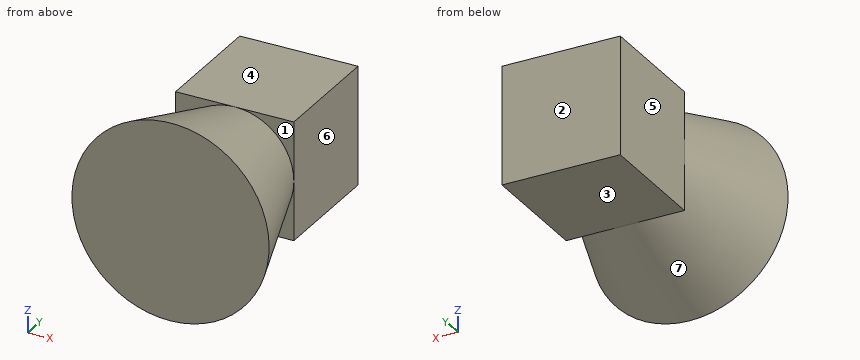
```python
from build123d import *

# Parameters (mm, degrees)
SKETCH_2_W      = 30
SKETCH_2_H      = 30
EXTRUDE_1_DEPTH = 30


with BuildPart() as part:
    # 草图2 → 凸台-拉伸1 (new body)
    with BuildSketch(Plane(origin=(0, 0, 0), x_dir=(1, 0, 0), z_dir=(0, 1, 0))):
        Rectangle(SKETCH_2_W, SKETCH_2_H)
    extrude(amount=EXTRUDE_1_DEPTH)

    # 草图3 → 旋转1 (revolve)
    with BuildSketch(Plane.XY, mode=Mode.PRIVATE) as revolve_1_sk:
        Polygon((0, 0), (15, 0), (25, -30), (0, -30), align=None)
    revolve(revolve_1_sk.sketch.rotate(Axis((0, -30, 0), (0, 1, 0)), 90), axis=Axis((0, -30, 0), (0, 1, 0)))


solid = part.part
```
Geometry check sheet. Reference: the model listing, model coordinates, mm. Face numbers are marked on the shaded views. A direction names the side the tool comes from. Round coordinates to 2 decimals unless told otherwise and drop trailing zeros. Order: outer loops, then holes, each group sorted by start corner. A loop starts at its lowest first (then second) coordinate and runs counter-clockwise, first axis right, second up. Notation, with made-up numbers: (68.25, -16.75) - (118.25, -16.75) arc R8 cw to (118.25, -4.75) - close; hole circle Ø11 at (39.5, 22). An arc over 180 degrees is marked (long way). Use a Markdown table: item, result. Add a question column.
1) Set-up check for the marked faces 4, 5, 6 and 7: record each of +Z, -Z, +X, -X, +Y, -Y from which the full face is reachable in a straight line by a thin tool's end or side.
2) Gauge pin test, flat ends, axial feed: P1, Ø1.5, axis at x = -4.5, y = 9.5, coming from the +Z side; P2, Ø1, axis at x = 10.5, y = 11.5, coming from the -Z side; P3, Ø24, axis at y = 22, z = -2.5, coming from the +X side; P4, Ø1.5, axis at x = 19, y = -5, coming from the +Z side. Record the tip position at first contact, or that the pin passes through.
3) Section check B-B (y = -9.5). Record the cut outline in (x, z).
4) Section check A-A (y = 23). Record the cut outline in (x, z), then the cut area to 3 significant figures.
5) Mould release check, pull along Y, two halves, no side actions. Record for the marked faces 1, 2 and 3: released by +Y, released by -Y, zero draft, split by the parting line, or undercut.
6) Thickness scan on line 1 along X through (y, z) = (13, 14); line 2 along Z through (x, y) = (-13, -26.5). Record the ranges inside material, lowest first.
Established:
| question | item | result |
|---|---|---|
| 1 | face 4 | +Z, +X, -X, +Y |
| 1 | face 5 | +Z, -Z, -X, +Y |
| 1 | face 6 | +Z, -Z, +X, +Y |
| 1 | face 7 | none |
| 2 | P1 | z = 15 |
| 2 | P2 | z = -15 |
| 2 | P3 | x = 15 |
| 2 | P4 | through |
| 3 | outline | circle Ø36.33 at (0, 0) |
| 4 | outline | (-15, -15) - (15, -15) - (15, 15) - (-15, 15) - close |
| 4 | area | 900 mm2 |
| 5 | face 1 | undercut |
| 5 | face 2 | released by +Y |
| 5 | face 3 | zero draft |
| 6 | line 1 | -15 to 15 |
| 6 | line 2 | -19.98 to 19.98 |
